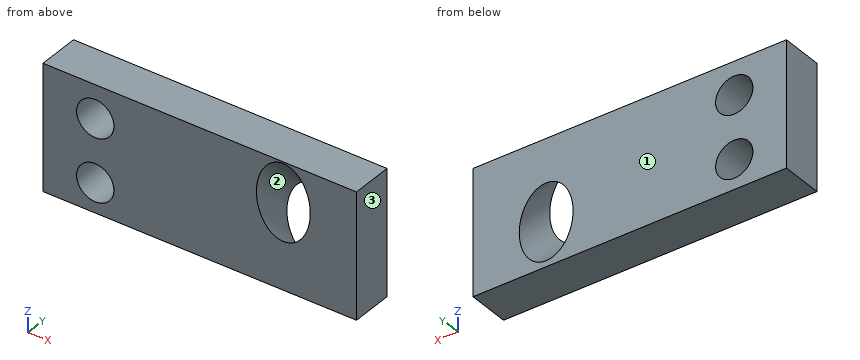
from build123d import *

# Parameters (mm, degrees)
SCHIZZO1_W                   = 30
SCHIZZO1_H                   = 12
SCHIZZO1_R                   = 1.785023435
ESTRUSIONE_ESTRUSIONE1_DEPTH = 4
SCHIZZO3_R                   = 2.575
TAGLIO_ESTRUSIONE2_DEPTH     = 25


with BuildPart() as part:
    # Schizzo1 → Estrusione-Estrusione1 (new body)
    with BuildSketch(Plane(origin=(0, 0, 0), x_dir=(1, 0, 0), z_dir=(0, 1, 0))):
        Rectangle(SCHIZZO1_W, SCHIZZO1_H)
        with Locations(Location((-10, 3.166569094, 0), (0, 0, 270))):
            Circle(SCHIZZO1_R, mode=Mode.SUBTRACT)
        with Locations(Location((-10, -2.833430906, 0), (0, 0, 270))):
            Circle(SCHIZZO1_R, mode=Mode.SUBTRACT)
    extrude(amount=ESTRUSIONE_ESTRUSIONE1_DEPTH)

    # Schizzo3 → Taglio-Estrusione2 (cut, symmetric)
    with BuildSketch(Plane(origin=(0, 2.9, -2.9), x_dir=(1, 0, 0), z_dir=(0, -0.7071067811865512, 0.7071067811865438))):
        with Locations(Location((8, 1.555634919, 0), (0, 0, 90))):
            Circle(SCHIZZO3_R)
    extrude(amount=TAGLIO_ESTRUSIONE2_DEPTH, both=True, mode=Mode.SUBTRACT)


solid = part.part
Source: CAD feature listing. Evaluate the final solid. Frame: model axes, mm. Face numbers are marked on the shaded views. Round coordinates to 2 decimals unless told otherwise and drop trailing zeros. Loops run counter-clockwise (first coordinate to the right, second up) from the corner with the lowest first, then second, coordinate; pieces in that order, holes last. Notation, with made-up numbers: (64.5, 10) - (71.5, 10) arc R3 cw to (71.5, 15) - close; hole circle Ø8 at (66, -2). An arc over 180 degrees is marked (long way). Write item = value, one per line. Start each with the question number.
Item 1: Material intervals for line 1 (Z direction, x = -9, y = 2.5); line 2 (X direction, y = 3.65, z = -2.5); line 3 (X direction, y = 2.95, z = 2.25), sorted ascending.
Item 2: Mould query, pull axis X, two halves, no side actions, for the marked faces 1, 2 and 3. Classes: released by +X, released by -X, zero draft, split by the parting line, or undercut.
Item 3: Section query C-C on y = 1.3. Count the separate pieces of the cut face and the enclosed holes in it, plus the area to 3 significant figures.
Item 4: Section query B-B on x = 10. Output: boundary loops of the cut face in (y, z), plus the area to 4 significant figures.
Item 5: Section query A-A on x = -10. Output: boundary loops of the cut face in (y, z), plus the area to 3 significant figures.
Item 6: First-contact query: pin 1 Ø3 at (x, z) = (-10, -3.17) entering from +Y. Flat tip, straight axial feed; report the tip coordinate or a pass-through.
Results list:
q1.line_1 = -6 to -4.65, -1.69 to 1.35, 4.31 to 6
q1.line_2 = -15 to -11.66, -8.34 to 5.53, 10.47 to 15
q1.line_3 = -15 to -11.69, -8.31 to 6.54, 9.46 to 15
q2.face_1 = zero draft
q2.face_2 = undercut
q2.face_3 = released by +X
q3.separate_pieces = 1
q3.enclosed_holes = 3
q3.area = 311 mm²
q4.outline = (0, -6) - (4, -6) - (4, -4.09) - (0, -0.09) - close; (0, 4.49) - (4, 0.49) - (4, 6) - (0, 6) - close
q4.area = 29.65 mm²
q5.outline = (0, -6) - (4, -6) - (4, -4.95) - (0, -4.95) - close; (0, -1.38) - (4, -1.38) - (4, 1.05) - (0, 1.05) - close; (0, 4.62) - (4, 4.62) - (4, 6) - (0, 6) - close
q5.area = 19.4 mm²
q6.pin_1 = through
